CAD build for the part. Positions are in the model's coordinates, mm. A direction names the side the tool comes from. Round coordinates to 2 decimals unless told otherwise and drop trailing zeros. Loops run counter-clockwise (first coordinate to the right, second up) from the corner with the lowest first, then second, coordinate; pieces in that order, holes last.
```python
from build123d import *

# Parameters (mm, degrees)
SKETCH1_R           = 1.5
SKETCH1_R_2         = 2.5
BOSS_EXTRUDE1_DEPTH = 3


with BuildPart() as part:
    # Sketch1 → Boss-Extrude1 (new body)
    with BuildSketch(Plane.XY):
        with BuildLine():
            Line((-32.5, 45), (32.5, 45))
            ThreePointArc((32.5, 45), (41.338834765, 41.338834765), (45, 32.5))
            Line((45, 32.5), (45, -32.5))
            ThreePointArc((45, -32.5), (41.338834765, -41.338834765), (32.5, -45))
            Line((32.5, -45), (32.5, -57.5))
            ThreePointArc((32.5, -57.5), (31.035533906, -61.035533906), (27.5, -62.5))
            Line((27.5, -62.5), (-27.5, -62.5))
            ThreePointArc((-27.5, -62.5), (-31.035533906, -61.035533906), (-32.5, -57.5))
            Line((-32.5, -57.5), (-32.5, -45))
            ThreePointArc((-32.5, -45), (-41.338834765, -41.338834765), (-45, -32.5))
            Line((-45, -32.5), (-45, 32.5))
            ThreePointArc((-45, 32.5), (-41.338834765, 41.338834765), (-32.5, 45))
        make_face()
        with Locations((-23, -8.2)):
            Circle(SKETCH1_R, mode=Mode.SUBTRACT)
        with Locations((23, -8.2)):
            Circle(SKETCH1_R, mode=Mode.SUBTRACT)
        with Locations((23, -51.8)):
            Circle(SKETCH1_R, mode=Mode.SUBTRACT)
        with Locations((-23, -51.8)):
            Circle(SKETCH1_R, mode=Mode.SUBTRACT)
        with Locations((-32.5, 32.5)):
            Circle(SKETCH1_R_2, mode=Mode.SUBTRACT)
        with Locations((32.5, 32.5)):
            Circle(SKETCH1_R_2, mode=Mode.SUBTRACT)
        with Locations((32.5, -32.5)):
            Circle(SKETCH1_R_2, mode=Mode.SUBTRACT)
        with Locations((-32.5, -32.5)):
            Circle(SKETCH1_R_2, mode=Mode.SUBTRACT)
    extrude(amount=BOSS_EXTRUDE1_DEPTH)


solid = part.part
```
Item 1: 3-axis set-ups, long thin cutter, end or side, ignore diameter. For faces 1 (the flat face through (-32.5, -51, 1)), 2 (the flat face through (45, 0, 1)): which of +Z, -Z, +X, -X, +Y, -Y reach the whole face in a straight line?
Answers follow:
face 1: +Z, -Z, -X, -Y
face 2: +Z, -Z, +X, +Y, -Y
Item 2: Two-plate mould, pull along X, no slides. Class faces 3 (the flat face through (32.5, -51, 1)), 4 (the cylindrical face through (-32.83, -30.02, 1.48)), 5 (the cylindrical face through (-41.241, -41.435, 1.479)), 6 (the cylindrical face through (21.89, -50.79, 1.48)): released by +X, released by -X, zero draft, split by the parting line, or undercut.
Answers follow:
face 3: released by +X
face 4: undercut
face 5: released by -X
face 6: undercut
Item 3: Cut at C-C, the plane y = -49. Give the cut face in (x, z).
Answers follow:
outline: (-32.5, 0) - (32.5, 0) - (32.5, 3) - (-32.5, 3) - close
Item 4: Cut at D-D, the plane x = 37.5. Give the cut face in (y, z).
Answers follow:
outline: (-43.96, 0) - (43.96, 0) - (43.96, 3) - (-43.96, 3) - close
Item 5: Flat gauge pin, fed straight in: P1, Ø1.5, axis at y = -54.5, z = 1.5, coming from the -X side. Where does the tip first touch, or does it go through?
Answers follow:
P1: stops at x = -32.5
Item 6: Cut at B-B, the plane z = 0.85. State how many separate pieces and enclosed holes the cut face has, plus the area to 3 significant figures.
Answers follow:
separate pieces: 1
enclosed holes: 8
area: 8,990 mm2
Item 7: Probe line 1 (Y direction, x = -23, z = 1.75); line 2 (X direction, y = -54, z = 0.4); line 3 (Y direction, x = 24, z = 1.45). List the from-to ranges inside material, lowest first.
Answers follow:
line 1: y = -62.5 to -53.3, -50.3 to -9.7, -6.7 to 45
line 2: x = -32.5 to 32.5
line 3: y = -62.5 to -52.92, -50.68 to -9.32, -7.08 to 45
Item 8: Cut at A-A, the plane x = -23. Give the cut face in (y, z), plus the area to 4 significant figures.
Answers follow:
outline: (-62.5, 0) - (-53.3, 0) - (-53.3, 3) - (-62.5, 3) - close; (-50.3, 0) - (-9.7, 0) - (-9.7, 3) - (-50.3, 3) - close; (-6.7, 0) - (45, 0) - (45, 3) - (-6.7, 3) - close
area: 304.5 mm2
